Input: part model. Units: mm. Frame: model coordinates. Face numbers are marked on the shaded views. A direction names the side the tool comes from. Round coordinates to 2 decimals unless told otherwise and drop trailing zeros. Order: outer loops, then holes, each group sorted by start corner. A loop starts at its lowest first (then second) coordinate and runs counter-clockwise, first axis right, second up. Notation, with made-up numbers: (-33.75, 43) -> (-11.75, 43) arc R34 ccw to (-11.75, 75) -> close; hole circle Ø9 at (61, 85). An arc over 180 degrees is marked (long way). Use a Markdown table: item, result.
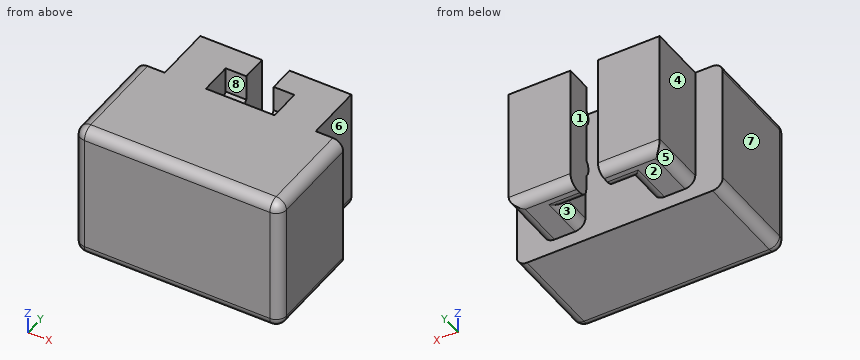
from build123d import *

# Parameters (mm, degrees)
SKETCH1_W            = 30
SKETCH1_H            = 20
BOSS_EXTRUDE1_DEPTH  = 15
BOSS_EXTRUDE2_DEPTH  = 18
SKETCH3_W            = 2.5
SKETCH3_H            = 0.5
BOSS_EXTRUDE3_DEPTH  = 3
FILLET1_R            = 1.5
FILLET1_OF_MIRROR1_R = 1.5
MIRROR2_START        = 5
MIRROR2_OUTLINE_W    = 8.45
MIRROR2_OUTLINE_H    = 18
MIRROR2_DEPTH        = 6
MIRROR2_START_2      = 2
MIRROR2_2_DEPTH      = 3
FILLET2_R            = 1.5


# Read off the part's stored shape, not the designer's step: Mirror2
with BuildPart() as part:
    # Sketch1 → Boss-Extrude1 (new body)
    with BuildSketch(Plane(origin=(0, 0, 0), x_dir=(1, 0, 0), z_dir=(0, 1, 0))):
        Rectangle(SKETCH1_W, SKETCH1_H)
    extrude(amount=BOSS_EXTRUDE1_DEPTH)

    # Sketch2 → Boss-Extrude2 (add)
    with BuildSketch(Plane.XY.offset(10)):
        Polygon((-11, 15), (-11, 23.45), (-2, 23.45), (-2, 19.7), (-5, 19.7), (-5, 15), align=None)
    extrude(amount=-BOSS_EXTRUDE2_DEPTH)

    # Sketch3 → Boss-Extrude3 (add)
    with BuildSketch(Plane(origin=(-5, 0, 0), x_dir=(0, 0, -1), z_dir=(1, 0, 0))):
        with Locations((-5, 19.45)):
            Rectangle(SKETCH3_W, SKETCH3_H)
    boss_extrude3 = extrude(amount=BOSS_EXTRUDE3_DEPTH)

    # Fillet1
    # the kernel refuses this fillet: 1.5 mm, written as the material it takes off along each edge
    with BuildSketch(Plane(origin=(-5, 19.2, 3.75), x_dir=(0, 1, 0), z_dir=(1, 0, 0))) as fillet1_piece_1:
        with BuildLine():
            CenterArc((1.5, 1.118033989), FILLET1_R, 180, 48.189685104)
            Line((0, 1.118033989), (-0.03, 1.118033989))
            Line((-0.03, 1.118033989), (-0.03, 0))
            Line((-0.03, 0), (0, -0.03))
            ThreePointArc((0, -0.03), (0.25, -0.03), (0.48, -0.02236068))
            Line((0.48, -0.02236068), (0.5, 0))
        make_face()
    extrude(amount=5.795084972, mode=Mode.SUBTRACT)
    with BuildSketch(Plane(origin=(-5, 19.2, 6.25), x_dir=(0, 1, 0), z_dir=(1, 0, 0))) as fillet1_piece_2:
        with BuildLine():
            CenterArc((1.5, -1.118033989), FILLET1_R, 131.810314896, 48.189685104)
            Line((0, -1.118033989), (-0.03, -1.118033989))
            Line((-0.03, -1.118033989), (-0.03, 0))
            Line((-0.03, 0), (0, 0.03))
            ThreePointArc((0, 0.03), (0.25, 0.03), (0.48, 0.02236068))
            Line((0.48, 0.02236068), (0.5, 0))
        make_face()
    extrude(amount=5.795084972, mode=Mode.SUBTRACT)

    # Mirror1: Boss-Extrude3 across plane
    add(boss_extrude3.mirror(Plane(origin=(0, 0, 1), x_dir=(1, 0, 0), z_dir=(0, 0, -1))))

    # Fillet1 of Mirror1
    # the kernel refuses this fillet: 1.5 mm, written as the material it takes off along each edge
    with BuildSketch(Plane(origin=(-5, 19.2, -1.75), x_dir=(0, 0, -1), z_dir=(1, 0, 0))) as fillet1_of_mirror1_piece_1:
        with BuildLine():
            CenterArc((1.118033989, 1.5), FILLET1_OF_MIRROR1_R, 221.810314896, 48.189685104)
            Line((0, 0.5), (-0.02236068, 0.48))
            ThreePointArc((-0.02236068, 0.48), (-0.03, 0.25), (-0.03, 0))
            Line((-0.03, 0), (0, -0.03))
            Line((0, -0.03), (1.118033989, -0.03))
            Line((1.118033989, -0.03), (1.118033989, 0))
        make_face()
    extrude(amount=5.795084972, mode=Mode.SUBTRACT)
    with BuildSketch(Plane(origin=(-5, 19.2, -4.25), x_dir=(0, 1, 0), z_dir=(1, 0, 0))) as fillet1_of_mirror1_piece_2:
        with BuildLine():
            CenterArc((1.5, 1.118033989), FILLET1_OF_MIRROR1_R, 180, 48.189685104)
            Line((0, 1.118033989), (-0.03, 1.118033989))
            Line((-0.03, 1.118033989), (-0.03, 0))
            Line((-0.03, 0), (0, -0.03))
            ThreePointArc((0, -0.03), (0.25, -0.03), (0.48, -0.02236068))
            Line((0.48, -0.02236068), (0.5, 0))
        make_face()
    extrude(amount=5.795084972, mode=Mode.SUBTRACT)

    # Mirror2 outline → Mirror2 (add)
    with BuildSketch(Plane.YZ.offset(MIRROR2_START)):
        with Locations((19.225, 1)):
            Rectangle(MIRROR2_OUTLINE_W, MIRROR2_OUTLINE_H)
    extrude(amount=MIRROR2_DEPTH)

    # Mirror2 2 outline → Mirror2 2 (add)
    with BuildSketch(Plane.YZ.offset(MIRROR2_START_2)):
        with BuildLine():
            Line((19.7, -4.25), (19.7, -8))
            Line((19.7, -8), (23.45, -8))
            Line((23.45, -8), (23.45, 10))
            Line((23.45, 10), (19.7, 10))
            Line((19.7, 10), (19.7, 6.25))
            ThreePointArc((19.7, 6.25), (19.330693606, 5.744338447), (19.2, 5.131966011))
            Line((19.2, 5.131966011), (19.2, 4.868033989))
            ThreePointArc((19.2, 4.868033989), (19.330693606, 4.255661553), (19.7, 3.75))
            Line((19.7, 3.75), (19.7, -1.75))
            ThreePointArc((19.7, -1.75), (19.330693606, -2.255661553), (19.2, -2.868033989))
            Line((19.2, -2.868033989), (19.2, -3.131966011))
            ThreePointArc((19.2, -3.131966011), (19.330693606, -3.744338447), (19.7, -4.25))
        make_face()
    extrude(amount=MIRROR2_2_DEPTH)

    # Fillet2
    fillet2_edges = [part.edges().sort_by_distance(p)[0] for p in [
        (-11, 19.225, -8),
        (-6.5, 23.45, -8),
        (-3.5, 19.7, -8),
        (-5, 17.35, -8),
        (0, 0, -10),
        (15, 0, 0),
        (0, 0, 10),
        (-15, 0, 0),
        (-15, 7.5, -10),
        (15, 7.5, -10),
        (15, 7.5, 10),
        (-15, 7.5, 10),
        (5, 17.35, -8),
        (3.5, 19.7, -8),
        (6.5, 23.45, -8),
        (11, 19.225, -8),
    ]]
    fillet(fillet2_edges, radius=FILLET2_R)


solid = part.part
1) Cut plane B-B on x = 3. Return loops of the section in (y, z).
Results found:
| item | result |
|---|---|
| outline | (0, -8.5) arc R1.5 ccw to (1.5, -10) -> (15, -10) -> (15, 10) -> (1.5, 10) arc R1.5 ccw to (0, 8.5) -> close; (19.2, -3.13) arc R1.5 ccw to (19.7, -4.25) -> (19.7, -6.5) arc R1.5 ccw to (21.2, -8) -> (21.95, -8) arc R1.5 ccw to (23.45, -6.5) -> (23.45, 10) -> (19.7, 10) -> (19.7, 6.25) arc R1.5 ccw to (19.2, 5.13) -> (19.2, 4.87) arc R1.5 ccw to (19.7, 3.75) -> (19.7, -1.75) arc R1.5 ccw to (19.2, -2.87) -> close |
2) Line query: L1, parallel to X at y = 19.25, z = 1.5; L2, parallel to Z at x = -9, y = 17.25; L3, parallel to Y at x = 1.25, z = 3.75. Output: solid intervals per line, ascending. Write a range as [from, to].
Results found:
| item | result |
|---|---|
| L1 | x = [-11, -5], [5, 11] |
| L2 | z = [-8, 10] |
| L3 | y = [0, 15] |
3) Pull-direction query (X, two-part tool) for the marked faces 6, 7 and 8; classes: +X half, -X half, draft (parallel to the pull), parting line (faces both ways), or undercut.
Results found:
| item | result |
|---|---|
| face 6 | +X half |
| face 7 | -X half |
| face 8 | undercut |
4) Pin query (flat end, axial travel): pin 1 Ø1.5 at (y, z) = (18.5, -5) entering from -X; pin 2 Ø4.5 at (y, z) = (21, -3) entering from +X; pin 3 Ø2 at (x, y) = (-7, 18.5) entering from -Z. Return the tip coordinate at first contact, or that it passes through.
Results found:
| item | result |
|---|---|
| pin 1 | stops at x = -11 |
| pin 2 | stops at x = 11 |
| pin 3 | stops at z = -8 |
5) Cut plane D-D on x = -1.5. Return loops of the section in (y, z), and give its area (3 significant figures).
Results found:
| item | result |
|---|---|
| outline | (0, -8.5) arc R1.5 ccw to (1.5, -10) -> (15, -10) -> (15, 10) -> (1.5, 10) arc R1.5 ccw to (0, 8.5) -> close |
| area | 299 mm² |
6) Set-up query: the marked faces 1, 2, 3, 4 and 5. Return all of +Z, -Z, +X, -X, +Y, -Y with unobstructed straight access to the full face (end or side cutting, diameter ignored); none if empty.
Results found:
| item | result |
|---|---|
| face 1 | +Z, -Z, +Y |
| face 2 | -Z, +X, -X, +Y |
| face 3 | -Z |
| face 4 | +Z, -Z, -X, +Y |
| face 5 | -Z, -X, +Y |
7) Cut plane A-A on y = 17.75. Return loops of the section in (x, z).
Results found:
| item | result |
|---|---|
| outline | (-11, -6.5) arc R1.5 ccw to (-9.5, -8) -> (-6.5, -8) arc R1.5 ccw to (-5, -6.5) -> (-5, 10) -> (-11, 10) -> close; (5, -6.5) arc R1.5 ccw to (6.5, -8) -> (9.5, -8) arc R1.5 ccw to (11, -6.5) -> (11, 10) -> (5, 10) -> close |
8) Cut plane C-C on z = 2.25. Return loops of the section in (x, y), and give its area (3 significant figures).
Results found:
| item | result |
|---|---|
| outline | (-15, 1.5) arc R1.5 ccw to (-13.5, 0) -> (13.5, 0) arc R1.5 ccw to (15, 1.5) -> (15, 15) -> (11, 15) -> (11, 23.45) -> (2, 23.45) -> (2, 19.7) -> (5, 19.7) -> (5, 15) -> (-5, 15) -> (-5, 19.7) -> (-2, 19.7) -> (-2, 23.45) -> (-11, 23.45) -> (-11, 15) -> (-15, 15) -> close |
| area | 573 mm² |
